Geometry: see drawing. Coordinates: mm, zero at the bounding-box minimum. Round coordinates to 2 decimals unless told otherwise and drop trailing zeros. Loops run counter-clockwise (first coordinate to the right, second up) from the corner with the lowest first, then second, coordinate; pieces in that order, holes last.
(1) Line query: line 1 (X direction, y = 2, z = 2.2); line 2 (Y direction, x = 1.8, z = 2). Output: solid intervals per line, ascending.
(2) First-contact query: pin 1 Ø0.8 at (x, z) = (2, 2) entering from +Y; pin 2 Ø1.5 at (x, y) = (2, 5) entering from +Z; pin 3 Ø0.7 at (y, z) = (9, 2) entering from +X; pin 4 Ø1.9 at (x, z) = (1, 1) entering from -Y. Flat tips, straight axial feed; report the tip coordinate or a pass-through.
(3) Cut plane A-A, the plane y = 6.75. Output: boundary loops of the cut face in (x, z).
(4) Draft query along X for the marked faces 1, 2 and 3. Return one class per face: released by +X, released by -X, zero draft, split by the parting line, or undercut.
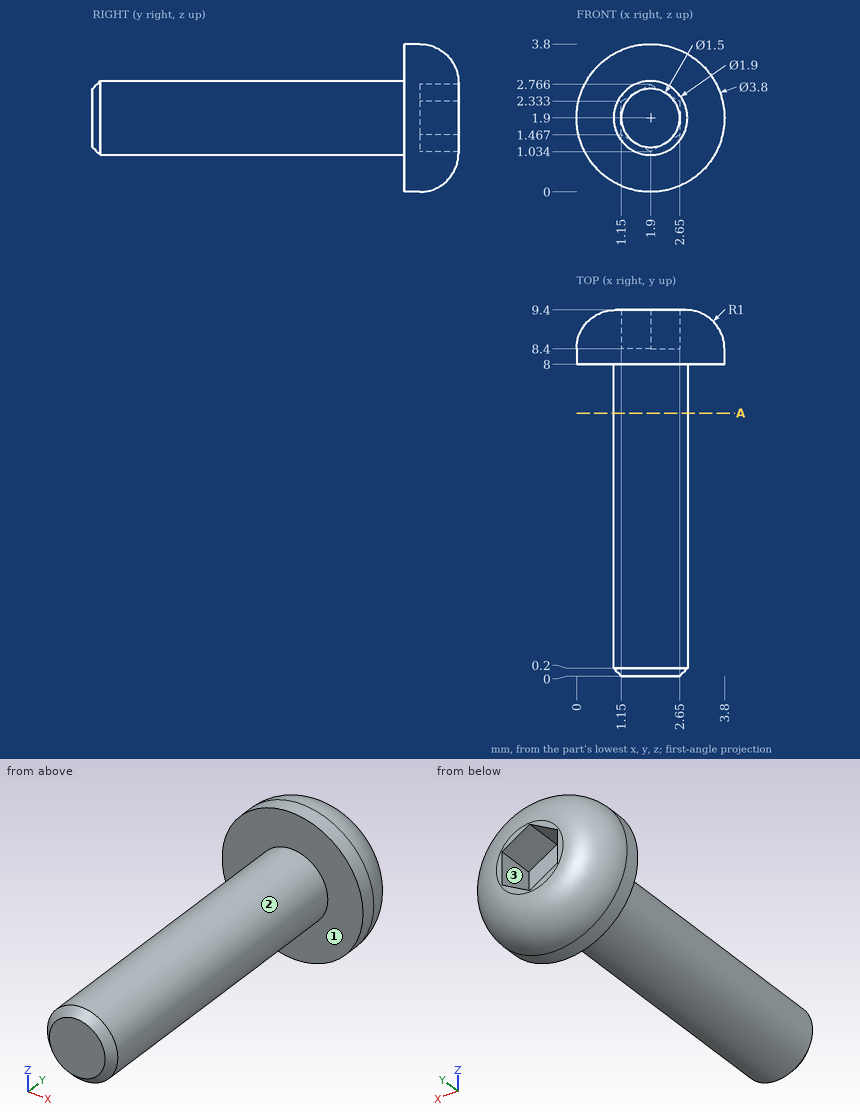
Reported:
1. line 1: x = 1 to 2.8
1. line 2: y = 0 to 8.4
2. pin 1: stops at y = 8.4
2. pin 2: stops at z = 2.85
2. pin 3: stops at x = 3.77
2. pin 4: stops at y = 0
3. outline: circle Ø1.9 at (1.9, 1.9)
4. face 1: zero draft
4. face 2: split by the parting line
4. face 3: undercut
